Design review of the part shown in the three views and the two pictorial views. Dimensions are in mm from the part's minimum x, y and z. A direction names the side the tool comes from. Round coordinates to 2 decimals unless told otherwise and drop trailing zeros. Write each loop counter-clockwise with the first axis right and the second up, starting at its lowest first coordinate (ties: lowest second). Pieces come first, ordered by that corner, then holes. Notation, with made-up numbers: (86, -1.5) -> (101, -1.5) arc R15 cw to (101, 18.5) -> close; hole circle Ø5 at (-14.5, 12.25). An arc over 180 degrees is marked (long way). Answer as a JSON object with one key per item and string values. Group by question number.
1) Insertion check: pin 1 Ø24 at (x, y) = (48.5, 36.5) entering from +Z; pin 2 Ø4 at (y, z) = (40, 69.5) entering from +X; pin 3 Ø8 at (x, y) = (74.5, 54) entering from +Z; pin 4 Ø1 at (y, z) = (12, 18.5) entering from +X. Each pin has a flat end and moves straight along its axis. Give the tip position at first contact, or say it passes through.
2) We need section B-B, the plane x = 56.5. Write out the cut boundary in (y, z).
3) Mouldability with a two-part tool opening along X and no side actions: class the marked faces 1, 2 and 3 as pulls with the +X half, pulls with the -X half, needs draft (parallel to the pull), parting line crosses it, or undercut.
4) We need section D-D, the plane z = 47. Write out the cut boundary in (x, y).
5) We need section C-C, the plane y = 43. Write out the cut boundary in (x, z), then the cut area to 3 significant figures.
6) We need section A-A, the plane z = 7.5. Write out the cut boundary in (x, y).
7) To check wall thickness, follow probe 1 along Y at (x, z) = (50, 23); probe 2 along Y at (x, z) = (95, 3.5); probe 3 along Z at (x, y) = (55, 5). State the ranges of each line that lie inside material, in increasing order. Write a range as [from, to].
8) Machinability: for the marked faces 4, 5, 6 and 7, which of the approach directions +Z, -Z, +X, -X, +Y, -Y give a long, thin tool a straight path to every point of the face, cutting with its end or side? Answer none if there is none.
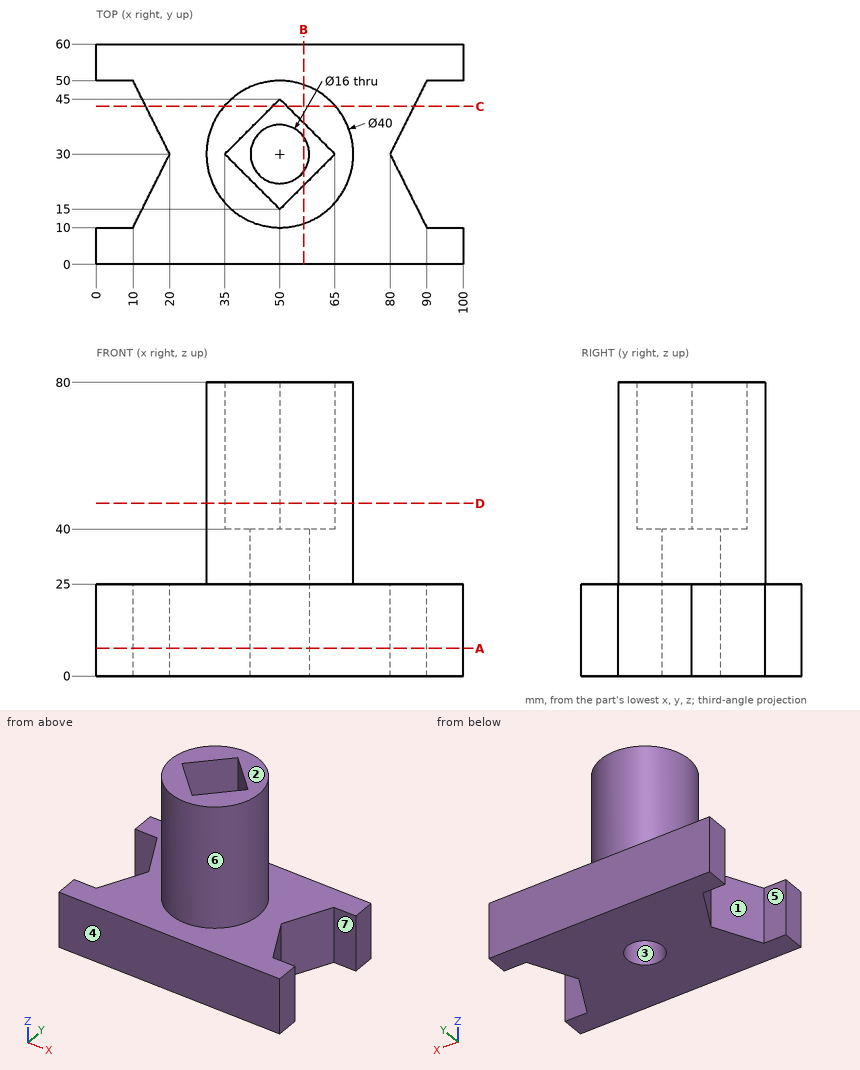
Here are the results:
{
 "1": {"pin 1": "stops at z = 80", "pin 2": "stops at x = 68.33", "pin 3": "stops at z = 25", "pin 4": "stops at x = 89.25"},
 "2": {"outline": "(0, 0) -> (25.34, 0) -> (25.34, 40) -> (21.5, 40) -> (21.5, 80) -> (11.09, 80) -> (11.09, 25) -> (0, 25) -> close; (34.66, 0) -> (60, 0) -> (60, 25) -> (48.91, 25) -> (48.91, 80) -> (38.5, 80) -> (38.5, 40) -> (34.66, 40) -> close"},
 "3": {"face 1": "pulls with the -X half", "face 2": "needs draft", "face 3": "undercut"},
 "4": {"outline": "circle Ø40 at (50, 30); hole (35, 30) -> (50, 15) -> (65, 30) -> (50, 45) -> close"},
 "5": {"outline": "(13.5, 0) -> (86.5, 0) -> (86.5, 25) -> (65.2, 25) -> (65.2, 80) -> (52, 80) -> (52, 40) -> (48, 40) -> (48, 80) -> (34.8, 80) -> (34.8, 25) -> (13.5, 25) -> close", "area": "3,340 mm^2"},
 "6": {"outline": "(0, 0) -> (100, 0) -> (100, 10) -> (90, 10) -> (80, 30) -> (90, 50) -> (100, 50) -> (100, 60) -> (0, 60) -> (0, 50) -> (10, 50) -> (20, 30) -> (10, 10) -> (0, 10) -> close; hole circle Ø16 at (50, 30)"},
 "7": {"probe 1": "y = [0, 22], [38, 60]", "probe 2": "y = [0, 10], [50, 60]", "probe 3": "z = [0, 25]"},
 "8": {"face 4": "+Z, -Z, +X, -X, -Y", "face 5": "+Z, -Z, -X", "face 6": "+Z", "face 7": "+Z, -Z, +X"}
}
